```python
from build123d import *

# Parameters (mm, degrees)
SKETCH2_R          = 1
CUT_EXTRUDE1_DEPTH = 4
SKETCH3_R          = 1
CUT_EXTRUDE2_DEPTH = 3


with BuildPart() as part:
    # Sketch1 → Revolve1 (revolve)
    with BuildSketch(Plane.XY):
        Polygon((0, 20.293987171), (0, 0), (0, -3.506012829), (1, -3.506012829), (1, -1.706012829), (9.5, -1.706012829), (11.5, 0.293987171), (11.5, 1.293987171), (11, 1.293987171), (11, 1.793987171), (11.5, 1.793987171), (11.5, 2.793987171), (9.5, 2.793987171), (9.5, 3.093987171), (11.5, 3.093987171), (11.5, 12.793987171), (7.5, 16.793987171), (1, 16.793987171), (1, 20.293987171), align=None)
        Polygon((2, 15.793987171), (7.085786438, 15.793987171), (10.5, 12.379773609), (10.5, 11.992676837), (1, 11.992676837), (1, 14.793987171), (2, 14.793987171), align=None, mode=Mode.SUBTRACT)
    revolve(axis=Axis((0, 20.293987171, 0), (0, -1, 0)))

    # Sketch2 → Cut-Extrude1 (cut)
    with BuildSketch(Plane(origin=(0, 16.793987171, 0), x_dir=(1, 0, 0), z_dir=(0, 1, 0))):
        with BuildLine():
            ThreePointArc((-4.999493877, -5.590622592), (-6.495190528, -3.75), (-7.341368127, -1.534377408))
            ThreePointArc((-7.341368127, -1.534377408), (-8.349114086, -1.551762877), (-9.294228634, -1.901923789))
            Line((-9.294228634, -1.901923789), (-15.450860687, -5.456456962))
            Line((-15.450860687, -5.456456962), (-12.450860687, -10.652609385))
            Line((-12.450860687, -10.652609385), (-6.294228634, -7.098076211))
            ThreePointArc((-6.294228634, -7.098076211), (-5.518423115, -6.454663459), (-4.999493877, -5.590622592))
        make_face()
        with BuildLine():
            ThreePointArc((-7.341368127, 1.534377408), (-6.495190528, 3.75), (-4.999493877, 5.590622592))
            ThreePointArc((-4.999493877, 5.590622592), (-5.518423115, 6.454663459), (-6.294228634, 7.098076211))
            Line((-6.294228634, 7.098076211), (-12.450860687, 10.652609385))
            Line((-12.450860687, 10.652609385), (-15.450860687, 5.456456962))
            Line((-15.450860687, 5.456456962), (-9.294228634, 1.901923789))
            ThreePointArc((-9.294228634, 1.901923789), (-8.349114086, 1.551762877), (-7.341368127, 1.534377408))
        make_face()
        with BuildLine():
            Line((-3, 16.109066347), (-3, 9))
            ThreePointArc((-3, 9), (-2.830690971, 8.006426336), (-2.341874249, 7.125))
            ThreePointArc((-2.341874249, 7.125), (0, 7.5), (2.341874249, 7.125))
            ThreePointArc((2.341874249, 7.125), (2.830690971, 8.006426336), (3, 9))
            Line((3, 9), (3, 16.109066347))
            Line((3, 16.109066347), (-3, 16.109066347))
        make_face()
        with BuildLine():
            ThreePointArc((6.294228634, 7.098076211), (5.518423115, 6.454663459), (4.999493877, 5.590622592))
            ThreePointArc((4.999493877, 5.590622592), (6.495190528, 3.75), (7.341368127, 1.534377408))
            ThreePointArc((7.341368127, 1.534377408), (8.349114086, 1.551762877), (9.294228634, 1.901923789))
            Line((9.294228634, 1.901923789), (15.450860687, 5.456456962))
            Line((15.450860687, 5.456456962), (12.450860687, 10.652609385))
            Line((12.450860687, 10.652609385), (6.294228634, 7.098076211))
        make_face()
        with BuildLine():
            ThreePointArc((9.294228634, -1.901923789), (8.349114086, -1.551762877), (7.341368127, -1.534377408))
            ThreePointArc((7.341368127, -1.534377408), (6.495190528, -3.75), (4.999493877, -5.590622592))
            ThreePointArc((4.999493877, -5.590622592), (5.518423115, -6.454663459), (6.294228634, -7.098076211))
            Line((6.294228634, -7.098076211), (12.450860687, -10.652609385))
            Line((12.450860687, -10.652609385), (15.450860687, -5.456456962))
            Line((15.450860687, -5.456456962), (9.294228634, -1.901923789))
        make_face()
        with BuildLine():
            ThreePointArc((2.341874249, -7.125), (0, -7.5), (-2.341874249, -7.125))
            ThreePointArc((-2.341874249, -7.125), (-2.830690971, -8.006426336), (-3, -9))
            Line((-3, -9), (-3, -16.109066347))
            Line((-3, -16.109066347), (3, -16.109066347))
            Line((3, -16.109066347), (3, -9))
            ThreePointArc((3, -9), (2.830690971, -8.006426336), (2.341874249, -7.125))
        make_face()
        with Locations((0, -4.5)):
            Circle(SKETCH2_R)
        with Locations((-4.5, 0)):
            Circle(SKETCH2_R)
        with Locations((0, 4.5)):
            Circle(SKETCH2_R)
        with Locations((4.5, 0)):
            Circle(SKETCH2_R)
    extrude(amount=-CUT_EXTRUDE1_DEPTH, mode=Mode.SUBTRACT)

    # Sketch3 → Cut-Extrude2 (cut)
    with BuildSketch(Plane.XZ.offset(1.706012829)):
        with Locations((0, -6)):
            Circle(SKETCH3_R)
        with Locations((0, 6)):
            Circle(SKETCH3_R)
        with Locations((8, 0)):
            Circle(SKETCH3_R)
        with Locations((-8, 0)):
            Circle(SKETCH3_R)
    extrude(amount=-CUT_EXTRUDE2_DEPTH, mode=Mode.SUBTRACT)


solid = part.part
```
Geometry check sheet. Reference: the model listing, model coordinates, mm. A direction names the side the tool comes from. Coordinates: 2 decimals unless noted, no trailing zeros. Write each loop counter-clockwise with the first axis right and the second up, starting at its lowest first coordinate (ties: lowest second). Pieces come first, ordered by that corner, then holes. Notation, with made-up numbers: M 6,-22.5 L 50,-22.5 A21 ccw 50,-14.5 Z; hole C -12.5,79 d6. An arc over 180 degrees is marked long. Answer as a JSON object with one key per item and string values.
1. Tool access check on faces 4 (the cylindrical face through (3.5, 16.3, 0)), 5 (the conical face through (-1.6, 15.6, -7.1)), 6 (the cylindrical face through (2.835, 15.117, 8.02)), 7 (the cylindrical face through (2.826, 15.117, -7.993)). Record the directions out of +Z, -Z, +X, -X, +Y, -Y that give a thin tool (end or side, any length) a straight path to the whole face; none if there is none.
Answers below:
{"face 4": "+Y", "face 5": "none", "face 6": "+Z, +Y", "face 7": "-Z, +Y"}
2. Go/stop test with flat-tipped pins: pin 1 Ø2 at (x, z) = (-8, -4.5) entering from +Y; pin 2 Ø10 at (y, z) = (8, -7) entering from +X; pin 3 Ø1.5 at (y, z) = (14, 8.5) entering from -X; pin 4 Ø1.5 at (y, z) = (14.5, 5) entering from +X. Record where each tip stops, or that it passes through.
Answers below:
{"pin 1": "stops at y = 12.79", "pin 2": "stops at x = 11.32", "pin 3": "stops at x = -7.34", "pin 4": "passes through"}
3. Section check D-D, the plane y = 9. Enter the section's corners in (x, z), plus the area to 3 significant figures.
Answers below:
{"outline": "C 0,0 d23", "area": "415 mm²"}
4. Draft check along X on faces 1 (the cylindrical face through (-1.5, 8, 11.4)), 2 (the flat face through (-1, 14.794, -1)), 3 (the conical face through (4.766, 14.822, 8.186)). Enter one of: released by +X, released by -X, zero draft, split by the parting line, or undercut.
Answers below:
{"face 1": "split by the parting line", "face 2": "undercut", "face 3": "released by +X"}
5. Section check B-B, the plane y = 17.25. Enter the section's corners in (x, z), plus the area to 3 significant figures.
Answers below:
{"outline": "C 0,0 d2", "area": "3.14 mm²"}
6. Section check A-A, the plane x = 0. Give the number of separate pieces and of enclosed holes in the cut face, plus the area to 3 significant figures.
Answers below:
{"separate pieces": "3", "enclosed holes": "0", "area": "331 mm²"}
7. Scan lines: L1, parallel to Y at x = 1.75, z = -4.25; L2, parallel to Z at x = 0, y = -0.9; L3, parallel to Y at x = -3.5, z = 9.25. Record each from-to range of solid material in increasing order.
Answers below:
{"L1": "y = -1.71 to 11.99, 15.79 to 16.79", "L2": "z = -10.31 to -7, -5 to 5, 7 to 10.31", "L3": "y = -1.32 to 2.79, 3.09 to 11.99, 12.99 to 14.4"}
